The figure shows three views and two pictorial views of one solid part (mm, origin at its lowest corner). Answer the questions. Give positions to 0.01 mm unless a question says otherwise; leave off trailing zeros. Loops run counter-clockwise (first coordinate to the right, second up) from the corner with the lowest first, then second, coordinate; pieces in that order, holes last. Notation, with made-up numbers: M -8.5,-39 L 49.5,-39 A17 ccw 49.5,-14 Z; hole C 2,67 d9. An arc over 180 degrees is marked long. Answer as a JSON object with one key per item and string values. Group by question number.
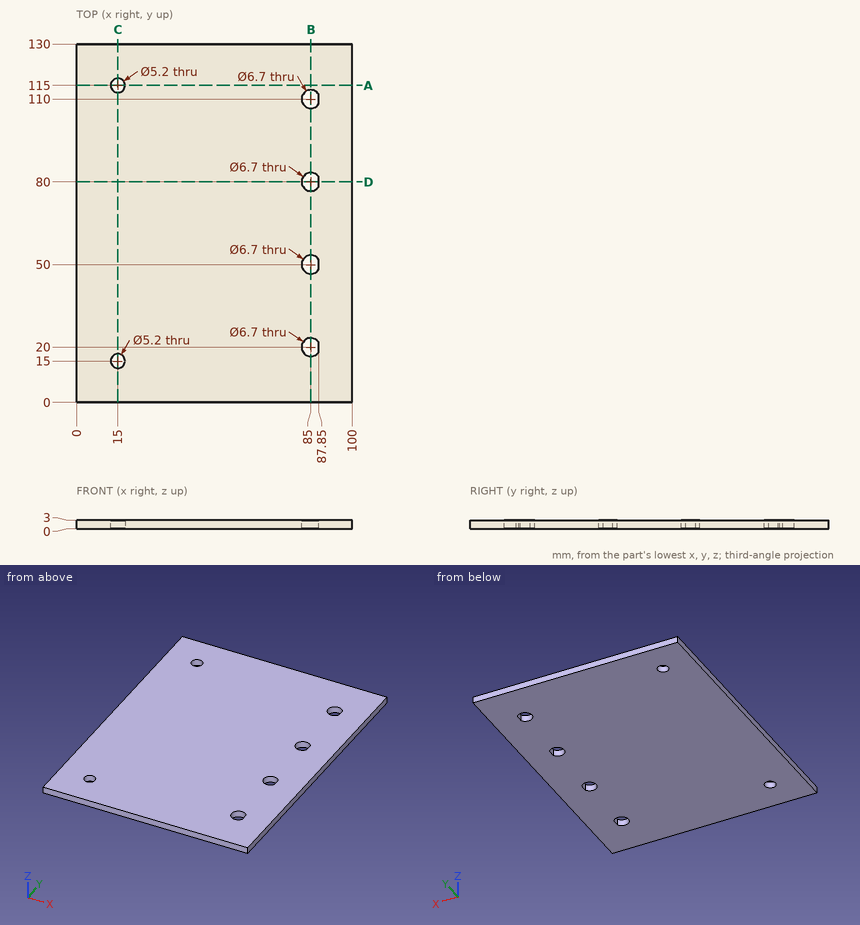
Item 1: A cutting plane is placed at C-C (x = 15). Determine the outline of the cut face in (y, z), and give its area (3 significant figures).
Item 2: A cutting plane is placed at B-B (x = 85). Determine the outline of the cut face in (y, z).
Item 3: A cutting plane is placed at A-A (y = 115). Determine the outline of the cut face in (x, z).
Item 4: A cutting plane is placed at D-D (y = 80). Determine the outline of the cut face in (x, z), and give its area (3 significant figures).
Item 5: Find the intervals of material crossed by probe 1 along Y at (x, z) = (85, 2.2); probe 2 along X at (y, z) = (50, 0.85); probe 3 along Y at (x, z) = (86, 0.65), in increasing order. Write a range as [from, to].
The answers:
{
 "1": {"outline": "M 0,0 L 12.4,0 L 12.4,3 L 0,3 Z; M 17.6,0 L 112.4,0 L 112.4,3 L 17.6,3 Z; M 117.6,0 L 130,0 L 130,3 L 117.6,3 Z", "area": "359 mm^2"},
 "2": {"outline": "M 0,0 L 16.65,0 L 16.65,3 L 0,3 Z; M 23.35,0 L 46.65,0 L 46.65,3 L 23.35,3 Z; M 53.35,0 L 76.65,0 L 76.65,3 L 53.35,3 Z; M 83.35,0 L 106.65,0 L 106.65,3 L 83.35,3 Z; M 113.35,0 L 130,0 L 130,3 L 113.35,3 Z"},
 "3": {"outline": "M 0,0 L 12.4,0 L 12.4,3 L 0,3 Z; M 17.6,0 L 100,0 L 100,3 L 17.6,3 Z"},
 "4": {"outline": "M 0,0 L 81.65,0 L 81.65,3 L 0,3 Z; M 87.85,0 L 100,0 L 100,3 L 87.85,3 Z", "area": "281 mm^2"},
 "5": {"probe 1": "y = [0, 16.65], [23.35, 46.65], [53.35, 76.65], [83.35, 106.65], [113.35, 130]", "probe 2": "x = [0, 81.65], [87.85, 100]", "probe 3": "y = [0, 16.8], [23.2, 46.8], [53.2, 76.8], [83.2, 106.8], [113.2, 130]"}
}
